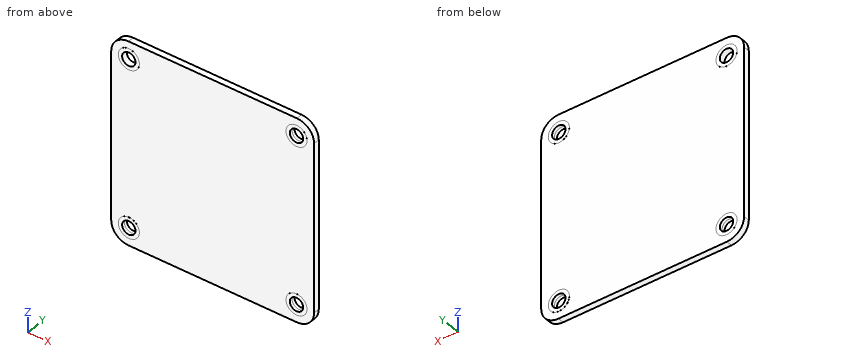
```python
from build123d import *

# Parameters (mm, degrees)
SKETCH1_R           = 1.755
BOSS_EXTRUDE1_DEPTH = 1.6
BOSS_EXTRUDE2_START = 0.8
SKETCH2_R           = 2.75
SKETCH2_R_2         = 1.75
BOSS_EXTRUDE2_DEPTH = 0.805


with BuildPart() as part:
    # Sketch1 → Boss-Extrude1 (new body)
    with BuildSketch(Plane(origin=(0, 0, 0), x_dir=(1, 0, 0), z_dir=(0, 1, 0))):
        with BuildLine():
            Line((22, -26.5), (-22, -26.5))
            ThreePointArc((-22, -26.5), (-25.181980515, -25.181980515), (-26.5, -22))
            Line((-26.5, -22), (-26.5, 22))
            ThreePointArc((-26.5, 22), (-25.181980515, 25.181980515), (-22, 26.5))
            Line((-22, 26.5), (22, 26.5))
            ThreePointArc((22, 26.5), (25.181980515, 25.181980515), (26.5, 22))
            Line((26.5, 22), (26.5, -22))
            ThreePointArc((26.5, -22), (25.181980515, -25.181980515), (22, -26.5))
        make_face()
        with Locations((-21.9, 21.9)):
            Circle(SKETCH1_R, mode=Mode.SUBTRACT)
        with Locations((21.9, 21.9)):
            Circle(SKETCH1_R, mode=Mode.SUBTRACT)
        with Locations((-21.9, -21.9)):
            Circle(SKETCH1_R, mode=Mode.SUBTRACT)
        with Locations((21.9, -21.9)):
            Circle(SKETCH1_R, mode=Mode.SUBTRACT)
    extrude(amount=BOSS_EXTRUDE1_DEPTH)

    # Sketch2 → Boss-Extrude2 (add, symmetric)
    with BuildSketch(Plane(origin=(0, 0, 0), x_dir=(1, 0, 0), z_dir=(0, 1, 0)).offset(BOSS_EXTRUDE2_START)):
        with Locations((-21.9, 21.9)):
            Circle(SKETCH2_R)
        with Locations((-21.9, 21.9)):
            Circle(SKETCH2_R_2, mode=Mode.SUBTRACT)
        with Locations((21.9, 21.9)):
            Circle(SKETCH2_R)
        with Locations((21.9, 21.9)):
            Circle(SKETCH2_R_2, mode=Mode.SUBTRACT)
        with Locations((21.9, -21.9)):
            Circle(SKETCH2_R)
        with Locations((21.9, -21.9)):
            Circle(SKETCH2_R_2, mode=Mode.SUBTRACT)
        with Locations((-21.9, -21.9)):
            Circle(SKETCH2_R)
        with Locations((-21.9, -21.9)):
            Circle(SKETCH2_R_2, mode=Mode.SUBTRACT)
    extrude(amount=BOSS_EXTRUDE2_DEPTH, both=True)


solid = part.part
```
Geometry: final body of the model. Coordinates: model frame, mm. Coordinates: 2 decimals unless noted, no trailing zeros. Order: outer loops, then holes, each group sorted by start corner. A loop starts at its lowest first (then second) coordinate and runs counter-clockwise, first axis right, second up. Notation, with made-up numbers: M 37,-1.75 L 88,-1.75 A22 ccw 88,17.25 Z; hole C 36.5,50 d6. An arc over 180 degrees is marked long. Answer in a Markdown table with one row per item. Add a question column.
Q1. Section query A-A on y = 1.25. Return the cut outline in (x, z).
Q2. Contact query for a flat-ended pin moving along its axis: P1, Ø6, axis at x = -6.5, z = 3.5, coming from the +Y side. Output: stop coordinate, or through.
Q3. Line query: L1, parallel to Z at x = 21.9, y = 0.4; L2, parallel to Y at x = 12.5, z = 4. Output: solid intervals per line, ascending.
Completed:
| question | item | result |
|---|---|---|
| 1 | outline | M -26.5,-22 A4.5 ccw -22,-26.5 L 22,-26.5 A4.5 ccw 26.5,-22 L 26.5,22 A4.5 ccw 22,26.5 L -22,26.5 A4.5 ccw -26.5,22 Z; hole C -21.9,-21.9 d3.5; hole C -21.9,21.9 d3.5; hole C 21.9,-21.9 d3.5; hole C 21.9,21.9 d3.5 |
| 2 | P1 | stops at y = 1.6 |
| 3 | L1 | z = -26.5 to -23.65, -20.15 to 20.15, 23.65 to 26.5 |
| 3 | L2 | y = 0 to 1.6 |
